Here's how the part is built. I have some questions about the finished solid (model axes, mm). A direction names the side the tool comes from. Round coordinates to 2 decimals unless told otherwise and drop trailing zeros. Order: outer loops, then holes, each group sorted by start corner. A loop starts at its lowest first (then second) coordinate and runs counter-clockwise, first axis right, second up. Notation, with made-up numbers: (-6.5, 6.25) - (39.5, 6.25) arc R23 cw to (39.5, 19.25) - close; hole circle Ø4 at (-37.5, 0). An arc over 180 degrees is marked (long way). Answer as a JSON object with one key per item and string values.
```python
from build123d import *

# Parameters (mm, degrees)
SKETCH2_R           = 1.5748
BOSS_EXTRUDE1_DEPTH = 3.175
SKETCH5_W           = 24.098
SKETCH5_H           = 3.175
BOSS_EXTRUDE2_DEPTH = 19.05
SKETCH7_W           = 1
SKETCH7_H           = 6.842
BOSS_EXTRUDE3_DEPTH = 3.175
SKETCH8_W           = 1
SKETCH8_H           = 3.175
BOSS_EXTRUDE4_DEPTH = 19.05
SKETCH9_W           = 3.175
SKETCH9_H           = 11.85042952
BOSS_EXTRUDE5_DEPTH = 10
CUT_EXTRUDE1_DEPTH  = 33.332180825


with BuildPart() as part:
    # Sketch2 → Boss-Extrude1 (new body)
    with BuildSketch(Plane.XY):
        Polygon((4.395213829, 10.321811953), (4.395213829, 7.827388121), (4.395213829, -1.438404904), (-11.860786171, -1.438404904), (-11.860786171, -8.280404904), (12.237213829, -8.280404904), (12.237213829, 12.658595096), (7.697213829, 12.658595096), (6.188170382, 12.658595096), (6.188170382, 10.321811953), align=None)
        with Locations((-9.320786171, -4.740404904)):
            Circle(SKETCH2_R, mode=Mode.SUBTRACT)
        with Locations((7.697213829, 8.213595096)):
            Circle(SKETCH2_R, mode=Mode.SUBTRACT)
    extrude(amount=BOSS_EXTRUDE1_DEPTH)

    # Sketch5 → Boss-Extrude2 (add)
    with BuildSketch(Plane(origin=(0, 0, 0), x_dir=(-1, 0, 0), z_dir=(0, 0, -1))):
        with Locations((-0.188213829, -9.867904904)):
            Rectangle(SKETCH5_W, SKETCH5_H)
    extrude(amount=-BOSS_EXTRUDE2_DEPTH)

    # Sketch7 → Boss-Extrude3 (add)
    with BuildSketch(Plane.XY.offset(3.175)):
        with Locations((-12.360786171, -4.859404904)):
            Rectangle(SKETCH7_W, SKETCH7_H)
    extrude(amount=-BOSS_EXTRUDE3_DEPTH)

    # Sketch8 → Boss-Extrude4 (add)
    with BuildSketch(Plane.XY.offset(19.05)):
        with Locations((-12.360786171, -9.867904904)):
            Rectangle(SKETCH8_W, SKETCH8_H)
    extrude(amount=-BOSS_EXTRUDE4_DEPTH)

    # Sketch9 → Boss-Extrude5 (add)
    with BuildSketch(Plane.XY.offset(3.175)):
        with Locations((8.404008836, -2.355190144)):
            Rectangle(SKETCH9_W, SKETCH9_H)
    extrude(amount=BOSS_EXTRUDE5_DEPTH)

    # Sketch10 → Cut-Extrude1 (cut, through all)
    with BuildSketch(Plane(origin=(9.991508836, 0, 0), x_dir=(0, 0, -1), z_dir=(1, 0, 0))):
        Polygon((-3.175, 3.570024616), (-13.175, -8.280404904), (-13.175, 3.570024616), align=None)
    extrude(amount=-CUT_EXTRUDE1_DEPTH, mode=Mode.SUBTRACT)


solid = part.part
```
1. Imagine slicing it at D-D (y = 9). List the corners of the cut face in (x, z) for me (3 decimals).
Responses:
{"outline": "(4.395, 0) - (6.333, 0) - (6.333, 3.175) - (4.395, 3.175) - close; (9.062, 0) - (12.237, 0) - (12.237, 3.175) - (9.062, 3.175) - close"}
2. If I drill on L1, parallel to Y at x = 7.5, z = 17; L2, parallel to X at y = 5.5, z = 2; L3, parallel to X at y = -4, z = 5.25, over which ranges is the centre line in solid material (lowest first)? Write a range as [from, to].
Responses:
{"L1": "[-11.46, -8.28]", "L2": "[4.4, 12.24]", "L3": "[6.82, 9.99]"}
3. Imagine slicing it at C-C (x = 1). List the corners of the cut face in (y, z) for me (3 decimals).
Responses:
{"outline": "(-11.455, 0) - (-1.438, 0) - (-1.438, 3.175) - (-8.28, 3.175) - (-8.28, 19.05) - (-11.455, 19.05) - close"}
4. Imagine slicing it at B-B (z = 2.75). List the corners of the cut face in (x, y) for me, plus the area to 3 significant figures.
Responses:
{"outline": "(-12.86, -11.46) - (12.24, -11.46) - (12.24, 12.66) - (6.19, 12.66) - (6.19, 10.32) - (4.4, 10.32) - (4.4, -1.44) - (-12.86, -1.44) - close; hole circle Ø3.15 at (-9.32, -4.74); hole circle Ø3.15 at (7.7, 8.21)", "area": "342 mm2"}
5. For faces 5 (the face through (2, -2, 3.175)), 6 (the face through (5, 10.322, 2)), 7 (the face through (6.817, -4, 7)), which set-ups out of +Z, -Z, +X, -X, +Y, -Y let a thin tool reach every point of the face, with its end or its side?
Responses:
{"face 5": "+Z, +Y", "face 6": "+Z, -Z, -X, +Y", "face 7": "+Z, -X, +Y"}
6. Imagine slicing it at A-A (x = -9.5). List the corners of the cut face in (y, z) for me (3 decimals).
Responses:
{"outline": "(-11.455, 0) - (-6.305, 0) - (-6.305, 3.175) - (-8.28, 3.175) - (-8.28, 19.05) - (-11.455, 19.05) - close; (-3.176, 0) - (-1.438, 0) - (-1.438, 3.175) - (-3.176, 3.175) - close"}
7. For P1, Ø5, axis at x = -3, z = 13, coming from the +Y side; P2, Ø8, axis at x = 6, z = 14, coming from the +Y side; P3, Ø1.9, axis at y = 12, z = 1.5, coming from the -X side, each with a flat end and sliding along its axis, tell me the tip position at first contact or that it passes through.
Responses:
{"P1": "y = -8.28", "P2": "y = -4.62", "P3": "x = 6.19"}
8. Thinking about a two-plate mould opening in X: for faces 1 (the face through (-12.861, -9, 8)), 2 (the face through (8.426, -2.272, 8.105)), 3 (the face through (-10.894, -4.671, 1.565)), 4 (the face through (7.492, 9.775, 1.565)), which applies, pulls with the +X half, pulls with the -X half, needs draft (parallel to the pull), parting line crosses it, or undercut?
Responses:
{"face 1": "pulls with the -X half", "face 2": "needs draft", "face 3": "undercut", "face 4": "undercut"}
